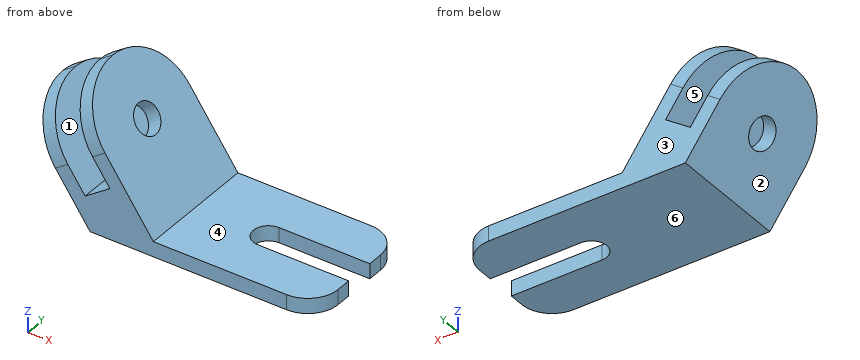
```python
from build123d import *

# Parameters (mm, degrees)
F1_DEPTH = 80
F2_R     = 39.99999
F4_DEPTH = 25
F5_R     = 20
F6_R     = 10
F7_DEPTH = 57.1


# Not quite as in the source:
# - a fillet or chamfer is up to 0.001 mm smaller than in the source, because OpenCascade refuses the exact size


with BuildPart() as f1:
    # F0 (on Front) → F1 (new body)
    with BuildSketch(Plane.XZ):
        Polygon((-121.122470571, 65.5321635431), (-75.236355663, 0), (74.763644337, 0), (74.763644337, 10), (-25.236355663, 10), (-33.4074474946, 10), (-88.3563887995, 88.4752209972), (-96.5479092424, 82.7394566337), (-62.1333230613, 33.5903339763), (-78.5163639471, 22.1188052493), (-112.9309501282, 71.2679279066), align=None)
    extrude(amount=F1_DEPTH)

    # F2 (radius 40 in the source; OpenCascade refuses exactly that, so slightly less here)
    f2_edges = [f1.edges().sort_by_distance(p)[0] for p in [
        (-92.452149, -80, 85.607339),
        (-117.02671, -80, 68.400046),
        (-92.452149, 0, 85.607339),
        (-117.02671, 0, 68.400046),
    ]]
    fillet(f2_edges, radius=F2_R)

    # F3 (on face) → F4 (cut)
    with BuildSketch(Plane.XY.offset(10)):
        with BuildLine():
            ThreePointArc((24.763644337, -40), (21.8347121489, -47.0710678119), (14.763644337, -50))
            Line((14.763644337, -50), (134.763644337, -50))
            Line((134.763644337, -50), (134.763644337, -30))
            Line((134.763644337, -30), (14.763644337, -30))
            ThreePointArc((14.763644337, -30), (21.8347121489, -32.9289321881), (24.763644337, -40))
        make_face()
        with BuildLine():
            ThreePointArc((14.763644337, -30), (4.763644337, -40), (14.763644337, -50))
            Line((14.763644337, -50), (14.763644337, -30))
        make_face()
        with BuildLine():
            Line((14.763644337, -30), (14.763644337, -50))
            ThreePointArc((14.763644337, -50), (21.8347121489, -47.0710678119), (24.763644337, -40))
            ThreePointArc((24.763644337, -40), (21.8347121489, -32.9289321881), (14.763644337, -30))
        make_face()
    extrude(amount=-F4_DEPTH, mode=Mode.SUBTRACT)

    # F5
    f5_edges = [f1.edges().sort_by_distance(p)[0] for p in [
        (74.763644, 0, 5),
        (74.763644, -80, 5),
    ]]
    fillet(f5_edges, radius=F5_R)

    # F6 (on face) → F7 (cut)
    with BuildSketch(Plane(origin=(-17.7182706335, 0, -12.4064666616), x_dir=(0, 1, 0), z_dir=(0.8191520443, 0, 0.5735764364))):
        with Locations((-40, 83.1538007652)):
            Circle(F6_R)
    extrude(amount=-F7_DEPTH, mode=Mode.SUBTRACT)


solid = f1.part
```
The model under review builds one solid part; all positions refer to its coordinate system, in mm. Face numbers are marked on the shaded views. A direction names the side the tool comes from. Round coordinates to 2 decimals unless told otherwise and drop trailing zeros. Write each loop counter-clockwise with the first axis right and the second up, starting at its lowest first coordinate (ties: lowest second). Pieces come first, ordered by that corner, then holes.
(1) We need section B-B on y = -8.5. Give the boundary of the cut face in (x, z) (3 decimals).
(2) We need section D-D on y = -54. Give the boundary of the cut face in (x, z), and give its area (3 significant figures).
(3) Insertion check: pin 1 (1.5 mm diameter, centred on y = -52, z = 35.5, fed in from +X); pin 2 (24 mm diameter, centred on x = 7.5, y = -27, fed in from +Z); pin 3 (3 mm diameter, centred on y = -56, z = 33, fed in from -X). Each pin has a flat end and moves straight along its axis. Give the tip position at first contact, or say it passes through.
(4) Mouldability with a two-part tool opening along X and no side actions: class the marked faces 1, 2 and 3 as +X half, -X half, draft (parallel to the pull), parting line (faces both ways), or undercut.
(5) Machinability: for the marked faces 4, 5 and 6, which of the approach directions +Z, -Z, +X, -X, +Y, -Y give a long, thin tool a straight path to every point of the face, cutting with its end or side? Answer none if there is none.
(6) We need section A-A on x = 37. Give the boundary of the cut face in (y, z).
(7) We need section C-C on x = -37. Give the boundary of the cut face in (y, z).
(8) Wall thickness on L1, parallel to Z at x = 17, y = -8; L2, parallel to Z at x = -63, y = -73; L3, parallel to X at y = -37.5, z = 64: over which ranges is each line inside the solid? List them lowest first.
Findings below:
1. outline: (-112.32, 52.96) - (-75.236, 0) - (71.127, 0) - (71.127, 10) - (-33.407, 10) - (-79.553, 75.903) - (-87.745, 70.168) - (-62.133, 33.59) - (-78.516, 22.119) - (-104.128, 58.696) - close
2. outline: (-119.67, 63.46) - (-75.24, 0) - (74.76, 0) - (74.76, 10) - (-33.41, 10) - (-86.91, 86.4) - (-95.1, 80.67) - (-62.13, 33.59) - (-78.52, 22.12) - (-111.48, 69.2) - close
2. area: 3,560 mm2
3. pin 1: stops at x = -50.74
3. pin 2: stops at z = 10
3. pin 3: stops at x = -99.39
4. face 1: undercut
4. face 2: -X half
4. face 3: draft
5. face 4: +Z, +X, +Y, -Y
5. face 5: +Y, -Y
5. face 6: -Z, +X, -X, +Y, -Y
6. outline: (-80, 0) - (-50, 0) - (-50, 10) - (-80, 10) - close; (-30, 0) - (0, 0) - (0, 10) - (-30, 10) - close
7. outline: (-80, 0) - (0, 0) - (0, 15.13) - (-80, 15.13) - close
8. L1: z = 0 to 10
8. L2: z = 0 to 32.98, 34.83 to 52.26
8. L3: x = -120.05 to -107.84, -83.43 to -71.22
